from build123d import *

# Parameters (mm, degrees)
EXTRUDE_1_DEPTH     = 14.3
SKETCH_2_R          = 1.75
CUT_EXTRUDE_1_DEPTH = 15.3
SKETCH_3_R          = 4
EXTRUDE_2_DEPTH     = 4
EXTRUDE_START       = -10
SKETCH_4_R          = 0.5
EXTRUDE_3_DEPTH     = 80


with BuildPart() as part:
    # 草圖1 → 填料-伸長1 (new body)
    with BuildSketch(Plane(origin=(0, 0, 0), x_dir=(1, 0, 0), z_dir=(0, 1, 0))):
        with BuildLine():
            Line((2, 0), (29.3, 0))
            ThreePointArc((29.3, 0), (30.714213562, 0.585786438), (31.3, 2))
            Line((31.3, 2), (31.3, 17.6))
            Line((31.3, 17.6), (0, 17.6))
            Line((0, 17.6), (0, 2))
            ThreePointArc((0, 2), (0.585786438, 0.585786438), (2, 0))
        make_face()
    extrude(amount=EXTRUDE_1_DEPTH)

    # 草圖2 → 除料-伸長1 (cut, through all)
    with BuildSketch(Plane(origin=(0, 14.3, 0), x_dir=(1, 0, 0), z_dir=(0, 1, 0))):
        with Locations((27.8, 3.5)):
            Circle(SKETCH_2_R)
        with Locations((3.5, 12.1)):
            Circle(SKETCH_2_R)
    extrude(amount=-CUT_EXTRUDE_1_DEPTH, mode=Mode.SUBTRACT)

    # 草圖3 → 填料-伸長2 (add)
    with BuildSketch(Plane.XZ):
        with Locations((8.8, -6)):
            Circle(SKETCH_3_R)
    extrude(amount=EXTRUDE_2_DEPTH)

    # 草圖4 → 填料-伸長3 (add)
    with BuildSketch(Plane.ZY.offset(EXTRUDE_START)):
        with Locations((-6, -3.4)):
            Circle(SKETCH_4_R)
    extrude(amount=-EXTRUDE_3_DEPTH)


solid = part.part
Part model, mm, in its own coordinate system. Give positions to 0.01 mm unless a question says otherwise; leave off trailing zeros. Write each loop counter-clockwise with the first axis right and the second up, starting at its lowest first coordinate (ties: lowest second). Pieces come first, ordered by that corner, then holes.
1) Probe L1, parallel to X at y = 9.25, z = -12.1; L2, parallel to Z at x = 27.8, y = 7.25; L3, parallel to Z at x = 3.5, y = 5. List the from-to ranges inside material, lowest first.
Resolved:
L1: x = 0 to 1.75, 5.25 to 31.3
L2: z = -17.6 to -5.25, -1.75 to 0
L3: z = -17.6 to -13.85, -10.35 to 0
2) Cut at D-D on z = -3.5. Write the cut outline in (x, y), then the cut area to 3 significant figures.
Resolved:
outline: (0, 0) - (5.68, 0) - (5.68, -4) - (11.92, -4) - (11.92, 0) - (26.05, 0) - (26.05, 14.3) - (0, 14.3) - close; (29.55, 0) - (31.3, 0) - (31.3, 14.3) - (29.55, 14.3) - close
area: 423 mm2
3) Two-plate mould, pull along Z, no slides. Class faces 1 (the face through (29.417, 7.25, -2.83)), 2 (the face through (31.3, 7, -10)), 3 (the face through (30.7, 7.05, -0.57)), 4 (the face through (3.12, 7.25, -10.39)): released by +Z, released by -Z, zero draft, split by the parting line, or undercut.
Resolved:
face 1: undercut
face 2: zero draft
face 3: released by +Z
face 4: undercut
4) Cut at C-C on y = 10.25. Write the cut outline in (x, z).
Resolved:
outline: (0, -17.6) - (31.3, -17.6) - (31.3, -2) arc R2 ccw to (29.3, 0) - (2, 0) arc R2 ccw to (0, -2) - close; hole circle Ø3.5 at (3.5, -12.1); hole circle Ø3.5 at (27.8, -3.5)
5) Cut at A-A on x = 3.5. Write the cut outline in (y, z).
Resolved:
outline: (0, -17.6) - (14.3, -17.6) - (14.3, -13.85) - (0, -13.85) - close; (0, -10.35) - (14.3, -10.35) - (14.3, 0) - (0, 0) - close
6) Cut at B-B on x = 27.8. Write the cut outline in (y, z).
Resolved:
outline: circle Ø1 at (-3.4, -6); (0, -17.6) - (14.3, -17.6) - (14.3, -5.25) - (0, -5.25) - close; (0, -1.75) - (14.3, -1.75) - (14.3, 0) - (0, 0) - close
7) Pin check, flat tips, straight feed: pin 1 (8 mm diameter, centred on y = 1.5, z = -2, fed in from +X); pin 2 (5.5 mm diameter, centred on x = 3.5, z = -12.1, fed in from -Y); pin 3 (2 mm diameter, centred on x = 27.8, z = -3.5, fed in from -Y). Stop position of each tip, or through.
Resolved:
pin 1: stops at x = 31.3
pin 2: stops at y = 0
pin 3: passes through
